Print and shaded views of the part. All mm, measured from the part's lowest x, y and z. A direction names the side the tool comes from. Round coordinates to 2 decimals unless told otherwise and drop trailing zeros. Order: outer loops, then holes, each group sorted by start corner. A loop starts at its lowest first (then second) coordinate and runs counter-clockwise, first axis right, second up. Notation, with made-up numbers: (-30, -2) - (-17, -2) arc R37 ccw to (-17, 34) - close; hole circle Ø3 at (64.25, 64). An arc over 180 degrees is marked (long way). Return JSON: item names as keys, results as strings. Group by question number.
Item 1: Saw through at C-C on x = 1.75. List the corners of the cut face in (y, z), and give its area (3 significant figures).
Item 2: Tool access for the marked faces 4, 5, 6, 7 and 8: list every direction of +Z, -Z, +X, -X, +Y, -Y with a clear straight run to the whole face (end or side of a thin tool).
Item 3: Two-plate mould, pull along X, no slides. Class the marked faces 1, 2 and 3: released by +X, released by -X, zero draft, split by the parting line, or undercut.
Item 4: Saw through at D-D on y = 4.5. List the corners of the cut face in (x, z).
Item 5: Probe probe 1 along X at (y, z) = (3, 0.95); probe 2 along Y at (x, z) = (6, 4); probe 3 along X at (y, z) = (6.5, 3.05). List the from-to ranges inside material, lowest first.
Item 6: Drop flat-ended pins along their axis: pin 1 (1.5 mm diameter, centred on x = 4.5, z = 2.5, fed in from +Y); pin 2 (1.2 mm diameter, centred on x = 4, y = 5.5, fed in from -Z); pin 3 (1.2 mm diameter, centred on x = 3.5, y = 6, fed in from +Z). Give the stop position or say it passes through.
Item 7: Saw through at B-B on y = 3.25. List the corners of the cut face in (x, z).
Item 8: Saw through at A-A on z = 2.1. List the corners of the cut face in (x, y).
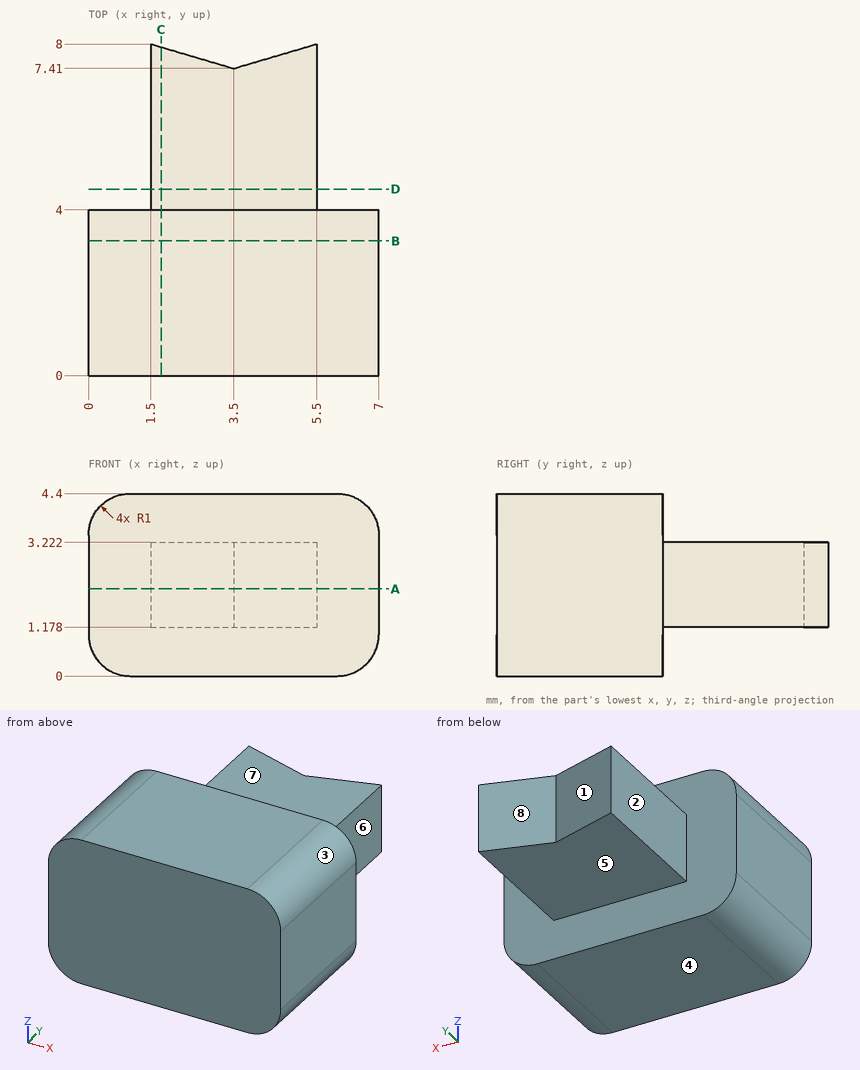
Filled in:
{
 "1": {"outline": "(0, 0) - (4, 0) - (4, 1.18) - (7.93, 1.18) - (7.93, 3.22) - (4, 3.22) - (4, 4.4) - (0, 4.4) - close", "area": "25.6 mm^2"},
 "2": {"face 4": "-Z, +X, -X, +Y, -Y", "face 5": "-Z, +X, -X, +Y", "face 6": "+Z, -Z, +X, +Y", "face 7": "+Z, +X, -X, +Y", "face 8": "+Z, -Z, +Y"},
 "3": {"face 1": "undercut", "face 2": "released by -X", "face 3": "released by +X"},
 "4": {"outline": "(1.5, 1.18) - (5.5, 1.18) - (5.5, 3.22) - (1.5, 3.22) - close"},
 "5": {"probe 1": "x = 0 to 7", "probe 2": "y = 0 to 4", "probe 3": "x = 1.5 to 5.5"},
 "6": {"pin 1": "stops at y = 7.93", "pin 2": "stops at z = 1.18", "pin 3": "stops at z = 3.22"},
 "7": {"outline": "(0, 1) arc R1 ccw to (1, 0) - (6, 0) arc R1 ccw to (7, 1) - (7, 3.4) arc R1 ccw to (6, 4.4) - (1, 4.4) arc R1 ccw to (0, 3.4) - close"},
 "8": {"outline": "(0, 0) - (7, 0) - (7, 4) - (5.5, 4) - (5.5, 8) - (3.5, 7.41) - (1.5, 8) - (1.5, 4) - (0, 4) - close"}
}
